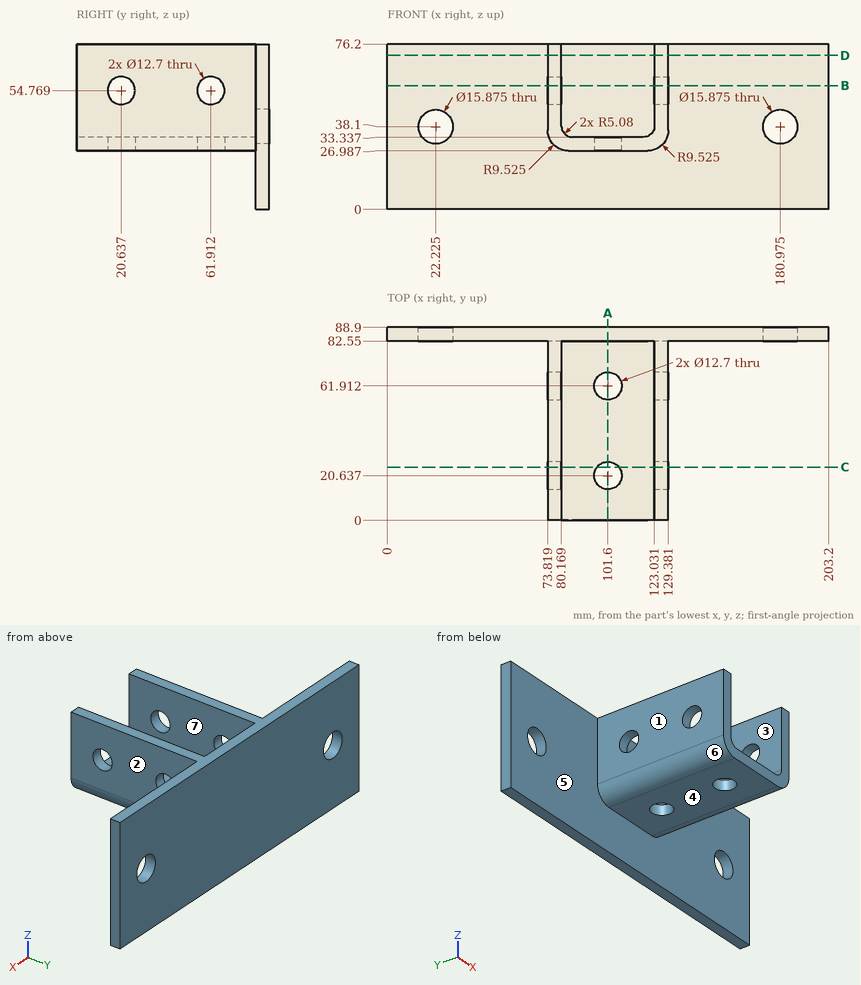
Verification items for this drawing (mm, ordinates from the low corner). A direction names the side the tool comes from. Round coordinates to 2 decimals unless told otherwise and drop trailing zeros. Loops run counter-clockwise (first coordinate to the right, second up) from the corner with the lowest first, then second, coordinate; pieces in that order, holes last. Notation, with made-up numbers: (71, 0) -> (108, 0) arc R16 cw to (108, 31) -> close; hole circle Ø3 at (42, 86). An arc over 180 degrees is marked (long way). Answer in a Markdown table with one row per item.
Q1. Sectioned sample at D-D on z = 71. Enter the section's corners in (x, y), then the cut area to 3 significant figures.
Data:
| item | result |
|---|---|
| outline | (0, 82.55) -> (73.82, 82.55) -> (73.82, 0) -> (80.17, 0) -> (80.17, 82.55) -> (123.03, 82.55) -> (123.03, 0) -> (129.38, 0) -> (129.38, 82.55) -> (203.2, 82.55) -> (203.2, 88.9) -> (0, 88.9) -> close |
| area | 2,340 mm^2 |
Q2. Thickness scan on L1, parallel to X at y = 85, z = 38; L2, parallel to X at y = 8.5, z = 70.5; L3, parallel to Z at x = 116.5, y = 25.5. Record the ranges inside material, lowest first.
Data:
| item | result |
|---|---|
| L1 | x = 0 to 14.29, 30.16 to 173.04, 188.91 to 203.2 |
| L2 | x = 73.82 to 80.17, 123.03 to 129.38 |
| L3 | z = 26.99 to 33.34 |
Q3. Set-up check for the marked faces 4, 5, 6 and 7: record each of +Z, -Z, +X, -X, +Y, -Y from which the full face is reachable in a straight line by a thin tool's end or side.
Data:
| item | result |
|---|---|
| face 4 | -Z, +X, -X, -Y |
| face 5 | -Z, -Y |
| face 6 | -Z, -X, -Y |
| face 7 | +Z, -Y |
Q4. Sectioned sample at A-A on x = 101.6. Enter the section's corners in (y, z).
Data:
| item | result |
|---|---|
| outline | (0, 26.99) -> (14.29, 26.99) -> (14.29, 33.34) -> (0, 33.34) -> close; (26.99, 26.99) -> (55.56, 26.99) -> (55.56, 33.34) -> (26.99, 33.34) -> close; (68.26, 26.99) -> (82.55, 26.99) -> (82.55, 0) -> (88.9, 0) -> (88.9, 76.2) -> (82.55, 76.2) -> (82.55, 33.34) -> (68.26, 33.34) -> close |
Q5. Release check for a two-part mould opening along X. For the marked faces 1, 2 and 3 record: released by +X, released by -X, zero draft, split by the parting line, or undercut.
Data:
| item | result |
|---|---|
| face 1 | released by -X |
| face 2 | released by +X |
| face 3 | undercut |
Q6. Sectioned sample at C-C on y = 24.5. Give the number of separate pieces and of enclosed holes in the cut face.
Data:
| item | result |
|---|---|
| separate pieces | 4 |
| enclosed holes | 0 |
Q7. Sectioned sample at B-B on z = 57. Enter the section's corners in (x, y).
Data:
| item | result |
|---|---|
| outline | (0, 82.55) -> (73.82, 82.55) -> (73.82, 67.86) -> (80.17, 67.86) -> (80.17, 82.55) -> (123.03, 82.55) -> (123.03, 67.86) -> (129.38, 67.86) -> (129.38, 82.55) -> (203.2, 82.55) -> (203.2, 88.9) -> (0, 88.9) -> close; (73.82, 0) -> (80.17, 0) -> (80.17, 14.69) -> (73.82, 14.69) -> close; (73.82, 26.58) -> (80.17, 26.58) -> (80.17, 55.97) -> (73.82, 55.97) -> close; (123.03, 0) -> (129.38, 0) -> (129.38, 14.69) -> (123.03, 14.69) -> close; (123.03, 26.58) -> (129.38, 26.58) -> (129.38, 55.97) -> (123.03, 55.97) -> close |
Q8. Go/stop test with flat-tipped pins: P1, Ø20, axis at y = 50.5, z = 49, coming from the -X side; P2, Ø4, axis at x = 133.5, z = 14.5, coming from the -Y side; P3, Ø20, axis at y = 45.5, z = 52, coming from the +X side. Record where each tip stops, or that it passes through.
Data:
| item | result |
|---|---|
| P1 | stops at x = 73.82 |
| P2 | stops at y = 82.55 |
| P3 | stops at x = 129.38 |
